```python
from build123d import *

# Parameters (mm, degrees)
SKETCH2_W          = 6
SKETCH2_H          = 5.216797091
CUT_EXTRUDE1_DEPTH = 69.439754529
CIRPATTERN1_COUNT  = 3


with BuildPart() as part:
    # Sketch1 → Revolve1 (revolve)
    with BuildSketch(Plane.XY, mode=Mode.PRIVATE) as revolve1_sk:
        Polygon((0, 30.125), (0, 42), (6, 42), (6, 34.485), (7, 34.485), (7, 34.985), (25, 34.985), (25, 34.485), (34, 34.485), (34, 30.125), align=None)
    revolve(revolve1_sk.sketch.rotate(Axis((0, 0, 0), (-1, 0, 0)), 90), axis=Axis((0, 0, 0), (-1, 0, 0)))

    # Sketch2 → Cut-Extrude1 (cut, through all)
    with BuildSketch(Plane.ZY):
        with Locations((0, 41.608398546)):
            Rectangle(SKETCH2_W, SKETCH2_H)
    cut_extrude1 = extrude(amount=-CUT_EXTRUDE1_DEPTH, mode=Mode.SUBTRACT)

    # CirPattern1: Cut-Extrude1 ×3 about axis
    cirpattern1_axis = Axis((0, 0, 0), (1, 0, 0))
    for i in range(1, CIRPATTERN1_COUNT):
        add(cut_extrude1.rotate(cirpattern1_axis, i * 360 / CIRPATTERN1_COUNT), mode=Mode.SUBTRACT)


solid = part.part
```
Work out the finished part from the listing and answer in its coordinate system (mm). A direction names the side the tool comes from. Coordinates: 2 decimals unless noted, no trailing zeros. Loops run counter-clockwise (first coordinate to the right, second up) from the corner with the lowest first, then second, coordinate; pieces in that order, holes last. Notation, with made-up numbers: M 45.5,73 L 90.5,73 A15 cw 90.5,82 Z; hole C 75,-24 d6. An arc over 180 degrees is marked long. Use CSV: the item, a comma, the result in double quotes. Start each with the question number.
(1) For faces 1 (the face through (3, 39, 0)), 2 (the face through (29.56, 20.98, 27.37)), 3 (the face through (7, 23, 26)), 4 (the face through (2.96, -19.54, -33.75)), determine the directions among +Z, -Z, +X, -X, +Y, -Y from which every point of the face is accessible in a straight line to the end or side of a thin tool.
(2) Find section D-D, the plane x = 26. Give the vertices of the cut face in (y, z) (3 decimals).
(3) Given pin 1 Ø3 at (x, z) = (24, 29.5) entering from +Y (3 decimals); pin 2 Ø6 at (x, z) = (28.5, 14) entering from -Y; pin 3 Ø6 at (x, z) = (17, 16) entering from +Y, each flat-ended and moving along its own axis, determine where each tip first touches the part or whether it passes through.
(4) For a pull along Z with two mould halves and no side action, classify faces 5 (the face through (2.96, -22.81, -33.51)), 6 (the face through (3.042, 20.501, 36.657)), 7 (the face through (2.96, -19.46, 33.8)) as +Z half, -Z half, draft (parallel to the pull), parting line (faces both ways), or undercut.
(5) Find section C-C, the plane x = 16. Give the vertices of the cut face in (y, z) (3 decimals), then the cut area to 3 significant figures.
(6) Find section A-A, the plane y = 0. Give the vertices of the cut face in (x, z) (3 decimals), then the cut area to 3 significant figures.
(7) Find section B-B, the plane z = 0. Give the vertices of the cut face in (x, y) (3 decimals).
(8) Consider line 1 (Y direction, x = 18.5, z = 0) (3 decimals); line 2 (X direction, y = -31, z = 21.5); line 3 (Y direction, x = 29, z = 11). Determine where each line is inside the solid, lowest interval first.
Recorded:
1,face 1,"+X, -X, +Y"
1,face 2,"+X"
1,face 3,"none"
1,face 4,"+X, -X"
2,outline,"C 0,0 d68.97; hole C 0,0 d60.25"
3,pin 1,"stops at y = 20.975"
3,pin 2,"stops at y = -32.68"
3,pin 3,"stops at y = 32.48"
4,face 5,"-Z half"
4,face 6,"+Z half"
4,face 7,"undercut"
5,outline,"C 0,0 d69.97; hole C 0,0 d60.25"
5,area,"994 mm^2"
6,outline,"M 0,-42 L 6,-42 L 6,-34.485 L 7,-34.485 L 7,-34.985 L 25,-34.985 L 25,-34.485 L 34,-34.485 L 34,-30.125 L 0,-30.125 Z; M 0,30.125 L 34,30.125 L 34,34.485 L 25,34.485 L 25,34.985 L 7,34.985 L 7,34.485 L 6,34.485 L 6,42 L 0,42 Z"
6,area,"405 mm^2"
7,outline,"M 0,-42 L 6,-42 L 6,-34.485 L 7,-34.485 L 7,-34.985 L 25,-34.985 L 25,-34.485 L 34,-34.485 L 34,-30.125 L 0,-30.125 Z; M 0,30.125 L 34,30.125 L 34,34.485 L 25,34.485 L 25,34.985 L 7,34.985 L 7,34.485 L 6,34.485 L 6,39 L 0,39 Z"
8,line 1,"y = -34.985 to -30.125, 30.125 to 34.985"
8,line 2,"x = 0 to 6"
8,line 3,"y = -32.68 to -28.04, 28.04 to 32.68"
